Geometry: final body of the model. Coordinates: model frame, mm. Round coordinates to 2 decimals unless told otherwise and drop trailing zeros. Write each loop counter-clockwise with the first axis right and the second up, starting at its lowest first coordinate (ties: lowest second). Pieces come first, ordered by that corner, then holes. Notation, with made-up numbers: M -31,24.25 L -15,24.25 A29 cw -15,45.25 Z; hole C -8,-19.5 d10. An arc over 180 degrees is marked long. Use one line per item in the form item = value. Start each with the question number.
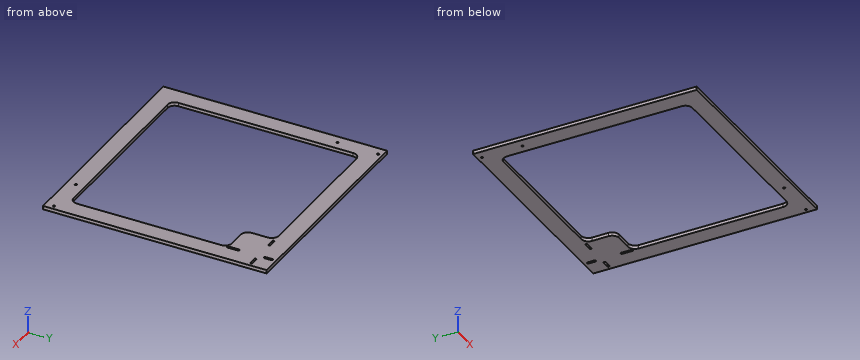
from build123d import *

# Parameters (mm, degrees)
F0_R     = 1.5
F1_DEPTH = 5


# Not quite as in the source:
# - ends of sketch curves that miss each other by under 0.0002 mm in the source are joined


with BuildPart() as f1:
    # F0 (on Top) → F1 (new body)
    with BuildSketch(Plane.XY):
        Polygon((-160, -160), (160, -160), (160, 110), (160, 160), (110, 160), (-160, 160), align=None)
        with Locations((96, -147.5)):
            Circle(F0_R, mode=Mode.SUBTRACT)
        with Locations((154, -147.5)):
            Circle(F0_R, mode=Mode.SUBTRACT)
        with Locations((-147.5, 96)):
            Circle(F0_R, mode=Mode.SUBTRACT)
        with Locations((-147.5, 154)):
            Circle(F0_R, mode=Mode.SUBTRACT)
        with BuildLine():
            ThreePointArc((135, -125), (132.0710678119, -132.0710678119), (125, -135))
            Line((125, -135), (-125, -135))
            ThreePointArc((-125, -135), (-132.0710678119, -132.0710678119), (-135, -125))
            Line((-135, -125), (-135, 125))
            ThreePointArc((-135, 125), (-132.0710678119, 132.0710678119), (-125, 135))
            Line((-125, 135), (81.5, 135))
            ThreePointArc((81.5, 135), (88.5710678119, 132.0710678119), (91.5, 125))
            Line((91.5, 125), (91.5, 101.5))
            ThreePointArc((91.5, 101.5), (94.4289321881, 94.4289321881), (101.5, 91.5))
            Line((101.5, 91.5), (125, 91.5))
            ThreePointArc((125, 91.5), (132.0710678119, 88.5710678119), (135, 81.5))
            Line((135, 81.5), (135, -125))
        make_face(mode=Mode.SUBTRACT)
        with BuildLine():
            ThreePointArc((133.4512195122, 105.877928352), (134.9512195122, 107.377928352), (136.4512195122, 105.877928352))
            Line((136.4512195122, 105.877928352), (136.499991364, 91.5050899728))
            ThreePointArc((136.499991364, 91.5050899728), (135.0025449901, 90.000002159), (133.5, 91.5))
            Line((133.5, 91.5), (133.451236778, 105.8728393094))
            ThreePointArc((133.451236778, 105.8728393094), (133.4512216704, 105.8753838124), (133.4512195122, 105.877928352))
        make_face(mode=Mode.SUBTRACT)
        with BuildLine():
            ThreePointArc((96, 133.5), (94.5, 135), (96, 136.5))
            Line((96, 136.5), (106, 136.5))
            ThreePointArc((106, 136.5), (107.5, 135), (106, 133.5))
            Line((106, 133.5), (96, 133.5))
        make_face(mode=Mode.SUBTRACT)
        with BuildLine():
            ThreePointArc((144, 133.5), (142.5, 135), (144, 136.5))
            Line((144, 136.5), (154, 136.5))
            ThreePointArc((154, 136.5), (155.5, 135), (154, 133.5))
            Line((154, 133.5), (144, 133.5))
        make_face(mode=Mode.SUBTRACT)
        with BuildLine():
            ThreePointArc((133.5, 154), (135, 155.5), (136.5, 154))
            Line((136.5, 154), (136.5, 144))
            ThreePointArc((136.5, 144), (135, 142.5), (133.5, 144))
            Line((133.5, 144), (133.5, 154))
        make_face(mode=Mode.SUBTRACT)
    extrude(amount=F1_DEPTH)


solid = f1.part
1. Ray query, probe 1 along Y at (x, z) = (-147.5, 3.55); probe 2 along Y at (x, z) = (154, 3.25). Return the intervals inside material, ascending.
2. Section query A-A (x = -73). Return loops of the section in (y, z), then the cut area to 3 significant figures.
3. Contact query for a flat-ended pin moving along its axis: pin 1 (2.5 mm diameter, centred on x = 154, y = -147.5, fed in from -Z). Output: stop coordinate, or through.
4. Section query C-C (z = 3.7). Give the number of separate pieces and of enclosed holes in the cut face, then the cut area to 3 significant figures.
Checks:
q1.probe_1 = -160 to 94.5, 97.5 to 152.5, 155.5 to 160
q1.probe_2 = -160 to -149, -146 to 133.5, 136.5 to 160
q2.outline = M -160,0 L -135,0 L -135,5 L -160,5 Z; M 135,0 L 160,0 L 160,5 L 135,5 Z
q2.area = 250 mm^2
q3.pin_1 = through
q4.separate_pieces = 1
q4.enclosed_holes = 9
q4.area = 31,300 mm^2
